Input: part model. Units: mm. Frame: model coordinates. Face numbers are marked on the shaded views. A direction names the side the tool comes from. Coordinates: 2 decimals unless noted, no trailing zeros. Write each loop counter-clockwise with the first axis right and the second up, starting at its lowest first coordinate (ties: lowest second). Pieces come first, ordered by that corner, then holes.
1) Set-up query: the marked faces 1 and 2. Return all of +Z, -Z, +X, -X, +Y, -Y with unobstructed straight access to the full face (end or side cutting, diameter ignored); none if empty.
2) Section query B-B (x = -82). Output: boundary loops of the cut face in (y, z), then the cut area to 3 significant figures.
3) Pin query (flat end, axial travel): pin 1 Ø4 at (y, z) = (30, -4.5) entering from +X; pin 2 Ø8 at (x, y) = (-16.5, 10.5) entering from +Z; pin 3 Ø23.5 at (x, y) = (-83, 7) entering from -Z. Return the tip coordinate at first contact, or that it passes through.
4) Line query: L1, parallel to Z at x = -82, y = -15.5; L2, parallel to X at y = 32, z = -7; L3, parallel to Z at x = -9, y = -4. Output: solid intervals per line, ascending.
5) Section query C-C (z = 17). Output: boundary loops of the cut face in (x, y), then the cut area to 3 significant figures.
6) Section query A-A (y = 2.5). Output: boundary loops of the cut face in (x, z), then the cut area to 3 significant figures.
from build123d import *

# Parameters (mm, degrees)
F0_W     = 82.8963629901
F0_H     = 57.0345446467
F1_DEPTH = 105.918
F3_DEPTH = 82.8973629901
F4_W     = 46.730304616
F4_H     = 11.7213707417
F5_DEPTH = 82.8973629901


with BuildPart() as f1:
    # F0 (on Right) → F1 (new body)
    with BuildSketch(Plane.YZ):
        with Locations((3.1172726303, -0.9236373007)):
            Rectangle(F0_W, F0_H)
    extrude(amount=-F1_DEPTH)

    # F2 (on face) → F3 (cut, through all)
    with BuildSketch(Plane.XZ.offset(38.3309088647)):
        Polygon((0, 27.5936350226), (-33.2005023956, 27.5936350226), (0, -29.4409096241), align=None)
    extrude(amount=-F3_DEPTH, mode=Mode.SUBTRACT)

    # F4 (on face) → F5 (cut, through all)
    with BuildSketch(Plane.XZ.offset(38.3309088647)):
        with Locations((-82.552847692, -23.5802242532)):
            Rectangle(F4_W, F4_H)
    extrude(amount=-F5_DEPTH, mode=Mode.SUBTRACT)


solid = f1.part
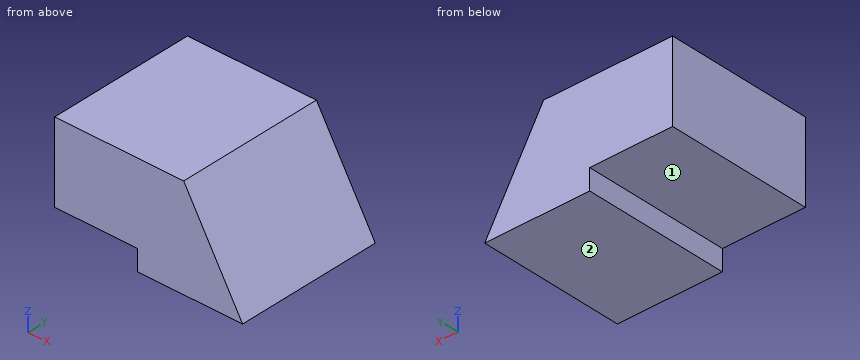
Answer:
1. face 1: -Z, -X, +Y, -Y
1. face 2: -Z, +X, -X, +Y, -Y
2. outline: (-38.33, -17.72) - (44.57, -17.72) - (44.57, 27.59) - (-38.33, 27.59) - close
2. area: 3,760 mm2
3. pin 1: stops at x = -13.35
3. pin 2: stops at z = 5.78
3. pin 3: stops at z = -17.72
4. L1: z = -17.72 to 27.59
4. L2: x = -105.92 to -13.06
4. L3: z = -29.44 to -13.98
5. outline: (-105.92, -38.33) - (-27.03, -38.33) - (-27.03, 44.57) - (-105.92, 44.57) - close
5. area: 6,540 mm2
6. outline: (-105.92, -17.72) - (-59.19, -17.72) - (-59.19, -29.44) - (0, -29.44) - (-33.2, 27.59) - (-105.92, 27.59) - close
6. area: 4,550 mm2
